Check sheet for the modelled part. Datum: model origin and axes. Units: mm. A direction names the side the tool comes from. Coordinates: 2 decimals unless noted, no trailing zeros. Order: outer loops, then holes, each group sorted by start corner. A loop starts at its lowest first (then second) coordinate and runs counter-clockwise, first axis right, second up.
from build123d import *

# Parameters (mm, degrees)
F1_DEPTH      = 38.1
F1_DEPTH_BACK = 38.1
F3_DEPTH      = 50.8
F3_DEPTH_BACK = 50.8
F4_R          = 10.332617
F4_R_2        = 9.383371
F5_DEPTH      = 73.557125


with BuildPart() as f1:
    # F0 (on Front) → F1 (new body, two sides)
    with BuildSketch(Plane.XZ) as f1_sk:
        with BuildLine():
            Line((-34.708198, 11.385217), (-77.499136, 11.385217))
            Line((-77.499136, 11.385217), (-77.499136, -62.170908))
            Line((-77.499136, -62.170908), (61.333679, -62.170908))
            Line((61.333679, -62.170908), (61.333679, 11.385217))
            Line((61.333679, 11.385217), (15.214554, 11.385217))
            ThreePointArc((15.214554, 11.385217), (-9.746822, -18.097968), (-34.708198, 11.385217))
        make_face()
    extrude(amount=F1_DEPTH)
    extrude(f1_sk.sketch, amount=-F1_DEPTH_BACK)

    # F2 (on Front) → F3 (join, two sides)
    with BuildSketch(Plane.XZ) as f3_sk:
        with BuildLine():
            ThreePointArc((15.214554, 11.385217), (-9.746822, -18.097968), (-34.708198, 11.385217))
            Line((-34.708198, 11.385217), (-56.103667, 11.385217))
            ThreePointArc((-56.103667, 11.385217), (-12.361825, -32.356624), (31.380016, 11.385217))
            Line((31.380016, 11.385217), (15.214554, 11.385217))
        make_face()
    extrude(amount=F3_DEPTH)
    extrude(f3_sk.sketch, amount=-F3_DEPTH_BACK)

    # F4 (on face) → F5 (cut, through all)
    with BuildSketch(Plane.XY.offset(11.385217)):
        with Locations((47.989529, 0)):
            Circle(F4_R)
        with Locations((-63.91912, 0)):
            Circle(F4_R_2)
    extrude(amount=-F5_DEPTH, mode=Mode.SUBTRACT)


solid = f1.part
(1) Cross-section at D-D (x = -59.5). Enter the section's corners in (y, z), and give its area (3 significant figures).
Filled in:
outline: (-38.1, -62.17) - (-8.28, -62.17) - (-8.28, 11.39) - (-38.1, 11.39) - close; (8.28, -62.17) - (38.1, -62.17) - (38.1, 11.39) - (8.28, 11.39) - close
area: 4,390 mm2
(2) Cross-section at B-B (z = 0.5). Enter the section's corners in (x, y).
Filled in:
outline: (-77.5, -38.1) - (-54.73, -38.1) - (-54.73, -50.8) - (-34.15, -50.8) - (-34.15, 50.8) - (-54.73, 50.8) - (-54.73, 38.1) - (-77.5, 38.1) - close; (14.66, -50.8) - (30, -50.8) - (30, -38.1) - (61.33, -38.1) - (61.33, 38.1) - (30, 38.1) - (30, 50.8) - (14.66, 50.8) - close; hole circle Ø18.77 at (-63.92, 0); hole circle Ø20.67 at (47.99, 0)
(3) Cross-section at A-A (y = 0). Enter the section's corners in (x, z).
Filled in:
outline: (-77.5, -62.17) - (-73.3, -62.17) - (-73.3, 11.39) - (-77.5, 11.39) - close; (-54.54, -62.17) - (37.66, -62.17) - (37.66, 11.39) - (15.21, 11.39) arc R25.31 cw (long way) to (-34.71, 11.39) - (-54.54, 11.39) - close; (58.32, -62.17) - (61.33, -62.17) - (61.33, 11.39) - (58.32, 11.39) - close
(4) Go/stop test with flat-tipped pins: P1, Ø1.5, axis at x = -1.5, z = -47, coming from the -Y side; P2, Ø17, axis at x = -63.92, y = 0, coming from the +Z side. Record where each tip stops, or that it passes through.
Filled in:
P1: stops at y = -38.1
P2: passes through
(5) Cross-section at C-C (z = -50). Enter the section's corners in (x, y), and give its area (3 significant figures).
Filled in:
outline: (-77.5, -38.1) - (61.33, -38.1) - (61.33, 38.1) - (-77.5, 38.1) - close; hole circle Ø18.77 at (-63.92, 0); hole circle Ø20.67 at (47.99, 0)
area: 9,970 mm2
(6) Thickness scan on probe 1 along X at (y, z) = (-25, 8); probe 2 along Y at (x, z) = (-64.5, -57); probe 3 along Y at (x, z) = (51, -37). Record the ranges inside material, lowest first.
Filled in:
probe 1: x = -77.5 to -35.04, 15.55 to 61.33
probe 2: y = -38.1 to -9.37, 9.37 to 38.1
probe 3: y = -38.1 to -9.88, 9.88 to 38.1
(7) Release check for a two-part mould opening along X. For faces 3 (the flat face through (-9, -38.1, -33)), 4 (the cylindrical face through (-9.13, 0.71, -18.09)), 5 (the cylindrical face through (-13.324, -44.361, -32.346)) record: +X half, -X half, draft (parallel to the pull), parting line (faces both ways), or undercut.
Filled in:
face 3: draft
face 4: undercut
face 5: parting line
(8) Tool access check on faces 1 (the cylindrical face through (37.667, 0.454, -24.878)), 2 (the cylindrical face through (-13.324, 44.361, -32.346)). Record the directions out of +Z, -Z, +X, -X, +Y, -Y that give a thin tool (end or side, any length) a straight path to the whole face; none if there is none.
Filled in:
face 1: +Z, -Z
face 2: -Z, +Y
